Here's how the part is built. I have some questions about the finished solid (model axes, mm). Face numbers are marked on the shaded views. Give positions to 0.01 mm unless a question says otherwise; leave off trailing zeros. Loops run counter-clockwise (first coordinate to the right, second up) from the corner with the lowest first, then second, coordinate; pieces in that order, holes last. Notation, with made-up numbers: M 78.25,59.25 L 97.25,59.25 A14 ccw 97.25,70.25 Z; hole C 45.5,54.5 d5. An arc over 180 degrees is marked long. Answer as CSV lines item,"result". Start each with the question number.
Item 1: I want a section at B-B on x = -39. List the corners of the cut face in (y, z) for me, plus the area to 3 significant figures.
Item 2: I want a section at A-A on y = 5. List the corners of the cut face in (x, z) for me (3 decimals), plus the area to 3 significant figures.
Item 3: I want a section at C-C on z = -43. List the corners of the cut face in (x, y) for me.
Item 4: I want a section at D-D on z = -123. List the corners of the cut face in (x, y) for me.
Item 5: Will these pins go through, and if not, where does the flat tip stop? P1, Ø5, axis at x = 15.5, y = 5, coming from the -Z side; P2, Ø21.5, axis at x = 98.5, z = -8.5, coming from the +Y side; P3, Ø11.5, axis at x = -95.5, z = -16, coming from the +Y side.
Item 6: If I drill on line 1 along Z through (x, y) = (-66.5, 7.75); line 2 along Z through (x, y) = (62, 7); line 3 along X through (y, z) = (3.5, -19), over which ranges is the centre line in solid material (lowest first)? Write a range as from..to.
Item 7: If we mould it in two halves opening along X, with no side actions, what happens to the marked faces 1 and 2? For each: released by +X, released by -X, zero draft, split by the parting line, or undercut.
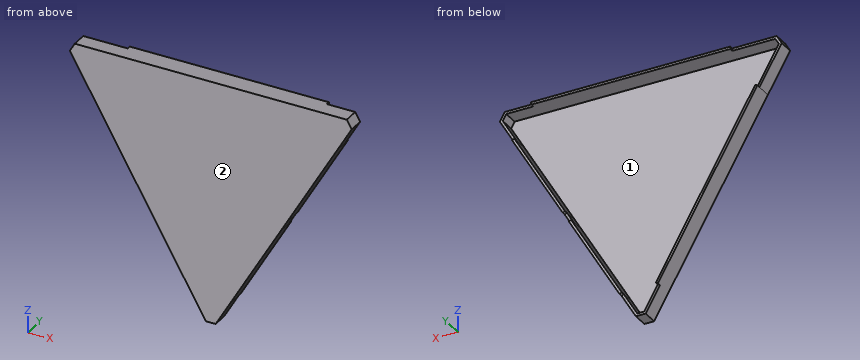
from build123d import *

# Parameters (mm, degrees)
BOSS_EXTRUDE1_DEPTH = 0.08
BOSS_EXTRUDE2_DEPTH = 12.46
SKETCH1_4_W         = 162.49
SKETCH1_4_H         = 2
BOSS_EXTRUDE3_DEPTH = 15.46


# Read off the part's stored shape, not the designer's step: Boss-Extrude2
with BuildPart() as part:
    # Sketch1 → Boss-Extrude1 (new body)
    with BuildSketch(Plane(origin=(0, 0, 0), x_dir=(1, 0, 0), z_dir=(0, 1, 0))):
        Polygon((-115, 0), (-111, -6.92820323), (111, -6.92820323), (115, 0), (15.625, 172.122549002), (13.892949192, 171.122549002), (2.845299462, 190.25763964), (-2.845299462, 190.25763964), (-13.892949192, 171.122549002), (-15.625, 172.122549002), align=None)
    extrude(amount=BOSS_EXTRUDE1_DEPTH)

    # Boss-Extrude2 outline → Boss-Extrude2 (add)
    with BuildSketch(Plane(origin=(0, 0, 0), x_dir=(1, 0, 0), z_dir=(0, 1, 0))):
        Polygon((15.625, 172.122549002), (4, 192.25763964), (-4, 192.25763964), (-15.625, 172.122549002), (-13.892949192, 171.122549002), (-2.845299462, 190.25763964), (2.845299462, 190.25763964), (13.892949192, 171.122549002), align=None)
        Polygon((62, 91.798692801), (57, 100.458946839), (55.267949192, 99.458946839), (60.267949192, 90.798692801), align=None)
        Polygon((-95.137949192, 30.402081141), (-96.87, 31.402081141), (-115, 0), (-111, -6.92820323), (-74.74, -6.92820323), (-74.74, -4.92820323), (-109.845299462, -4.92820323), (-112.690598923, 0), align=None)
        Polygon((115, 0), (103.375, 20.135090638), (101.642949192, 19.135090638), (112.690598923, 0), (109.845299462, -4.92820323), (87.75, -4.92820323), (87.75, -6.92820323), (111, -6.92820323), align=None)
    extrude(amount=BOSS_EXTRUDE2_DEPTH)

    # Sketch1<4> → Boss-Extrude3 (add)
    with BuildSketch(Plane(origin=(0, 0, 0), x_dir=(1, 0, 0), z_dir=(0, 1, 0))):
        Polygon((-15.625, 172.122549002), (-96.87, 31.402081141), (-95.137949192, 30.402081141), (-13.892949192, 171.122549002), align=None)
        with Locations((6.505, -5.92820323)):
            Rectangle(SKETCH1_4_W, SKETCH1_4_H)
        Polygon((57, 100.458946839), (15.625, 172.122549002), (13.892949192, 171.122549002), (55.267949192, 99.458946839), align=None)
        Polygon((101.642949192, 19.135090638), (103.375, 20.135090638), (62, 91.798692801), (60.267949192, 90.798692801), align=None)
    extrude(amount=BOSS_EXTRUDE3_DEPTH)


solid = part.part
Result:
1,outline,"M 0,-131.64 L 15.46,-131.64 L 15.46,-127.64 L 0.08,-127.64 L 0.08,4.93 L 15.46,4.93 L 15.46,6.93 L 0,6.93 Z"
1,area,"103 mm^2"
2,outline,"M -115,0 L -4,-192.258 L 4,-192.258 L 115,0 L 111,6.928 L -111,6.928 Z; hole M -112.691,0 L -2.845,-190.258 L 2.845,-190.258 L 112.691,0 L 109.845,4.928 L -109.845,4.928 Z"
2,area,"1,370 mm^2"
3,outline,"M -90.17,0 L 90.17,0 L 90.17,15.46 L 87.86,15.46 L 87.86,0.08 L -87.86,0.08 L -87.86,15.46 L -90.17,15.46 Z"
4,outline,"M -43.99,0 L 43.99,0 L 43.99,15.46 L 41.68,15.46 L 41.68,0.08 L -41.68,0.08 L -41.68,15.46 L -43.99,15.46 Z"
5,P1,"z = -176.67"
5,P2,"y = 12.46"
5,P3,"y = 0.08"
6,line 1,"-84..-80, 4.93..6.93"
6,line 2,"-91.8..-87.8, 4.93..6.93"
6,line 3,"-104.03..-101.72, 101.72..104.03"
7,face 1,"undercut"
7,face 2,"zero draft"
